The model under review builds one solid part; all positions refer to its coordinate system, in mm. A direction names the side the tool comes from. Coordinates: 2 decimals unless noted, no trailing zeros. Write each loop counter-clockwise with the first axis right and the second up, starting at its lowest first coordinate (ties: lowest second). Pieces come first, ordered by that corner, then holes.
1) Add section A-A, the plane x = 11. State the section outline as (y, z) points, then the cut area to 3 significant figures.
2) For line 1 (Z direction, x = 9, y = 4); line 2 (Z direction, x = -7.5, y = 14.5); line 3 (X direction, y = 21.5, z = 18.5), list the stretches that pass through material, from the lowest coordinate up.
3) Add section D-D, the plane x = -6. State the section outline as (y, z) points, then the cut area to 3 significant figures.
4) For P1, Ø15.5, axis at y = -7.5, z = 17, coming from the -X side; P2, Ø1.7, axis at y = 0.5, z = 32, coming from the -X side; P3, Ø1.6, axis at y = -8.5, z = 33.5, coming from the +X side; P4, Ø8, axis at x = -10.5, z = 29.5, coming from the +Y side, all flat-tipped, find the tip position at first contact; note any pin that passes through.
5) Add section C-C, the plane z = 24.5. State the section outline as (x, y) points.
6) Add section B-B, the plane y = 22. State the section outline as (x, z) points.
7) Mouldability with a two-part tool opening along X and no side actions: class faces 4 (the flat face through (6, 0, 29.931)), 5 (the flat face through (18, 0, 34.931)), 6 (the flat face through (-3.388, 0, 33)) as released by +X, released by -X, zero draft, split by the parting line, or undercut.
8) Machinability: for faces 1 (the flat face through (1, 0, 10.935)), 2 (the cylindrical face through (-1.5, -0.4, 38.1)), 3 (the cylindrical face through (15.71, -0.35, 30.786)), which of the approach directions +Z, -Z, +X, -X, +Y, -Y give a long, thin tool a straight path to every point of the face, cutting with its end or side? Answer none if there is none.
from build123d import *

# Parameters (mm, degrees)
F1_DEPTH = 25


with BuildPart() as f1:
    # F0 (on Front) → F1 (new body, symmetric)
    with BuildSketch(Plane.XZ):
        with BuildLine():
            Line((16.612064, 32.930892), (16.612064, 34.930892))
            Line((16.612064, 34.930892), (16.612064, 39.930892))
            Line((16.612064, 39.930892), (2.962064, 39.930892))
            ThreePointArc((2.962064, 39.930892), (-1.528064, 38.07102), (-3.387936, 33.580892))
            Line((-3.387936, 33.580892), (-3.387936, 31.430892))
            ThreePointArc((-3.387936, 31.430892), (-2.948596, 30.370232), (-1.887936, 29.930892))
            Line((-1.887936, 29.930892), (13.612064, 29.930892))
            ThreePointArc((13.612064, 29.930892), (15.733384, 30.809572), (16.612064, 32.930892))
        make_face()
        with BuildLine():
            Line((22.335033, 10.934645), (-20.985033, 10.934645))
            ThreePointArc((-20.985033, 10.934645), (-25.475161, 9.074773), (-27.335033, 4.584645))
            Line((-27.335033, 4.584645), (-27.335033, -4.584645))
            ThreePointArc((-27.335033, -4.584645), (-25.475161, -9.074773), (-20.985033, -10.934645))
            Line((-20.985033, -10.934645), (20.985033, -10.934645))
            ThreePointArc((20.985033, -10.934645), (25.475161, -9.074773), (27.335033, -4.584645))
            Line((27.335033, -4.584645), (27.335033, 10.934645))
            Line((27.335033, 10.934645), (22.335033, 10.934645))
        make_face()
        with BuildLine():
            Line((22.335033, 30.433444), (22.335033, 10.934645))
            Line((22.335033, 10.934645), (27.335033, 10.934645))
            Line((27.335033, 10.934645), (27.335033, 30.433444))
            ThreePointArc((27.335033, 30.433444), (25.109878, 36.602568), (19.459069, 39.930892))
            Line((19.459069, 39.930892), (16.612064, 39.930892))
            Line((16.612064, 39.930892), (16.612064, 34.930892))
            Line((16.612064, 34.930892), (18.907292, 34.930892))
            ThreePointArc((18.907292, 34.930892), (21.380409, 33.26083), (22.335033, 30.433444))
        make_face()
    extrude(amount=F1_DEPTH, both=True)


solid = f1.part
Geometry results:
1. outline: (-25, -10.93) - (25, -10.93) - (25, 10.93) - (-25, 10.93) - close; (-25, 29.93) - (25, 29.93) - (25, 39.93) - (-25, 39.93) - close
1. area: 1,590 mm2
2. line 1: z = -10.93 to 10.93, 29.93 to 39.93
2. line 2: z = -10.93 to 10.93
2. line 3: x = 22.34 to 27.34
3. outline: (-25, -10.93) - (25, -10.93) - (25, 10.93) - (-25, 10.93) - close
3. area: 1,090 mm2
4. P1: stops at x = -25.29
4. P2: stops at x = -3.39
4. P3: stops at x = 27.07
4. P4: passes through
5. outline: (22.34, -25) - (27.34, -25) - (27.34, 25) - (22.34, 25) - close
6. outline: (-27.34, -4.58) arc R6.35 ccw to (-20.99, -10.93) - (20.99, -10.93) arc R6.35 ccw to (27.34, -4.58) - (27.34, 30.43) arc R9.66 ccw to (19.46, 39.93) - (2.96, 39.93) arc R6.35 ccw to (-3.39, 33.58) - (-3.39, 31.43) arc R1.5 ccw to (-1.89, 29.93) - (13.61, 29.93) arc R3 ccw to (16.61, 32.93) - (16.61, 34.93) - (18.91, 34.93) arc R4.66 cw to (22.34, 30.43) - (22.34, 10.93) - (-20.99, 10.93) arc R6.35 ccw to (-27.34, 4.58) - close
7. face 4: zero draft
7. face 5: undercut
7. face 6: released by -X
8. face 1: -X, +Y, -Y
8. face 2: +Z, -X, +Y, -Y
8. face 3: +Y, -Y
